For this review, take the finished solid that the model builds, in its own axes (mm). A direction names the side the tool comes from. Coordinates: 2 decimals unless noted, no trailing zeros. Order: outer loops, then holes, each group sorted by start corner. A loop starts at its lowest first (then second) coordinate and runs counter-clockwise, first axis right, second up. Notation, with made-up numbers: (87, 11.25) -> (135, 11.25) arc R20 cw to (135, 50.25) -> close; hole circle Ø3 at (-34.5, 23.25). An arc over 180 degrees is marked (long way). Return JSON: item names as keys, results as strings. Group by question number.
Item 1: For line 1 along Z through (x, y) = (-17, 8.5); line 2 along Z through (x, y) = (0.5, 12); line 3 along Y through (x, z) = (0.5, 99.5), list the stretches that pass through material, from the lowest coordinate up.
Item 2: Draft analysis for pull direction X (two halves, no side actions). For faces 1 (the flat face through (0, 25, 97)), 2 (the flat face through (0.21, -15.28, 64.566)), 3 (the cylindrical face through (28, -34, 60)), 4 (the cylindrical face through (-21.445, 30.07, 130.979)), state which applies: +X half, -X half, draft (parallel to the pull), parting line (faces both ways), or undercut.
Item 3: Take a section at C-C (z = 35). Write out the cut boundary in (x, y), then the cut area to 3 significant figures.
Item 4: Take a section at A-A (y = 18). Write out the cut boundary in (x, z), then the cut area to 3 significant figures.
Item 5: Insertion check: pin 1 (7 mm diameter, centred on x = 0, z = 110, fed in from -Y); pin 2 (12 mm diameter, centred on y = 20.5, z = 17, fed in from +X); pin 3 (4 mm diameter, centred on x = -17, y = -4, fed in from +Z); pin 4 (6 mm diameter, centred on x = -1.5, z = 107, fed in from -Y). Each pin has a flat end and moves straight along its axis. Give the tip position at first contact, or say it passes through.
Item 6: Machinability: for faces 5 (the flat face through (15, -24, 67)), 6 (the flat face through (0, 15, 103)), 7 (the cylindrical face through (-3.47, -15.62, 26.17)), 8 (the flat face through (0, 35, 94)), which of the approach directions +Z, -Z, +X, -X, +Y, -Y give a long, thin tool a straight path to every point of the face, cutting with its end or side? Answer none if there is none.
Item 7: Take a section at D-D (x = -18.5). Write out the cut boundary in (y, z).
```python
from build123d import *

# Parameters (mm, degrees)
F0_R      = 16
F1_DEPTH  = 50
F4_R      = 3
F5_W      = 30
F5_H      = 40
F6_DEPTH  = 20
F8_DEPTH  = 15
F9_DEPTH  = 20
F11_W     = 60
F11_H     = 10
F12_DEPTH = 70
F13_R     = 29.99999
F16_DEPTH = 10
F18_R     = 6
F19_DEPTH = 50
F20_R     = 5


# Not quite as in the source:
# - a fillet or chamfer is up to 0.001 mm smaller than in the source, because OpenCascade refuses the exact size


with BuildPart() as f1:
    # F0 (on Top) → F1 (new body)
    with BuildSketch(Plane.XY):
        Circle(F0_R)
    extrude(amount=F1_DEPTH)

    # F4
    f4_edges = [f1.edges().sort_by_distance(p)[0] for p in [
        (-16, 0, 0),
    ]]
    fillet(f4_edges, radius=F4_R)

    # F5 (on offset) → F6 (join)
    with BuildSketch(Plane.XY.offset(50)):
        with Locations((0, -15)):
            Rectangle(F5_W, F5_H)
    extrude(amount=F6_DEPTH)

    # F7 (on Right) → F8 (cut, symmetric)
    with BuildSketch(Plane.YZ):
        Polygon((5, 70), (0, 70), (-35, 70), (-35, 59.2820323028), align=None)
    extrude(amount=F8_DEPTH, both=True, mode=Mode.SUBTRACT)

    # F3 (on offset) → F9 (join)
    with BuildSketch(Plane.XY.offset(50)):
        Polygon((30, 35), (-30, 35), (-30, -35), (-15, -35), (-15, 5), (15, 5), (15, -35), (30, -35), align=None)
    extrude(amount=F9_DEPTH)

    # F11 (on offset) → F12 (join)
    with BuildSketch(Plane.XY.offset(70)):
        with Locations((0, 30)):
            Rectangle(F11_W, F11_H)
    extrude(amount=F12_DEPTH)

    # F13 (radius 30 in the source; OpenCascade refuses exactly that, so slightly less here)
    f13_edges = [f1.edges().sort_by_distance(p)[0] for p in [
        (-30, 30, 140),
        (30, 30, 140),
    ]]
    fillet(f13_edges, radius=F13_R)

    # F15 (on offset) → F16 (join)
    with BuildSketch(Plane.XZ.offset(-25)):
        with BuildLine():
            ThreePointArc((0, 100), (7.0710678119, 102.9289321881), (10, 110))
            ThreePointArc((10, 110), (-7.0710678119, 117.0710678119), (0, 100))
        make_face()
    extrude(amount=F16_DEPTH)

    # F18 (on offset) → F19 (cut)
    with BuildSketch(Plane.XZ.offset(-15)):
        with Locations((0, 110)):
            Circle(F18_R)
    extrude(amount=-F19_DEPTH, mode=Mode.SUBTRACT)

    # F20
    f20_edges = [f1.edges().sort_by_distance(p)[0] for p in [
        (-30, -35, 60),
        (30, -35, 60),
    ]]
    fillet(f20_edges, radius=F20_R)


solid = f1.part
```
Findings below:
{
 "1": {"line 1": "z = 50 to 70", "line 2": "z = 0 to 70", "line 3": "y = 25 to 35"},
 "2": {"face 1": "draft", "face 2": "undercut", "face 3": "+X half", "face 4": "-X half"},
 "3": {"outline": "circle Ø32 at (0, 0)", "area": "804 mm2"},
 "4": {"outline": "(-30, 50) -> (30, 50) -> (30, 70) -> (-30, 70) -> close; circle Ø20 at (0, 110); hole circle Ø12 at (0, 110)", "area": "1,400 mm2"},
 "5": {"pin 1": "passes through", "pin 2": "stops at x = 6.76", "pin 3": "stops at z = 70", "pin 4": "stops at y = 15"},
 "6": {"face 5": "+Z, -Y", "face 6": "+Z, +X, -X, -Y", "face 7": "-Z", "face 8": "+Z, -Z, +X, -X, +Y"},
 "7": {"outline": "(-35, 50) -> (35, 50) -> (35, 133.62) -> (25, 133.62) -> (25, 70) -> (-35, 70) -> close"}
}
